The model under review builds one solid part; all positions refer to its coordinate system, in mm. A direction names the side the tool comes from. Round coordinates to 2 decimals unless told otherwise and drop trailing zeros. Loops run counter-clockwise (first coordinate to the right, second up) from the corner with the lowest first, then second, coordinate; pieces in that order, holes last. Notation, with made-up numbers: (13.25, 52.25) - (30.25, 52.25) arc R21 ccw to (30.25, 77.25) - close; hole circle Ø5 at (23, 50). An arc over 180 degrees is marked (long way). Answer as CSV lines item,"result".
from build123d import *
from build123d.topology import SkipClean

# Parameters (mm, degrees)
BOSS_EXTRUDE1_DEPTH = 3
SKETCH2_R           = 1.5
CUT_EXTRUDE1_DEPTH  = 9.507546276
CUT_EXTRUDE2_DEPTH  = 9.507546276


with BuildPart() as part:
    # Sketch1 → Boss-Extrude1 (new body)
    with BuildSketch(Plane(origin=(0, 0, 0), x_dir=(1, 0, 0), z_dir=(0, 1, 0))):
        with BuildLine():
            Line((-4.905, 2.614492754), (4.905, 2.614492754))
            ThreePointArc((4.905, 2.614492754), (7.519492754, 0), (4.905, -2.614492754))
            Line((4.905, -2.614492754), (-4.905, -2.614492754))
            ThreePointArc((-4.905, -2.614492754), (-7.519492754, 0), (-4.905, 2.614492754))
        make_face()
    extrude(amount=BOSS_EXTRUDE1_DEPTH)

    # Sketch2 → Cut-Extrude1 (cut, through all)
    with BuildSketch(Plane(origin=(0, 3, 0), x_dir=(1, 0, 0), z_dir=(0, 1, 0))):
        with Locations(Location((-4.905, 0, 0), (0, 0, 270))):
            Circle(SKETCH2_R)
        with Locations(Location((4.905, 0, 0), (0, 0, 270))):
            Circle(SKETCH2_R)
    extrude(amount=-CUT_EXTRUDE1_DEPTH, mode=Mode.SUBTRACT)

    # Sketch3 → Cut-Extrude2 (cut, through all)
    with SkipClean():  # the faces are left unmerged after this step: merging them gives an invalid solid
        with BuildSketch(Plane(origin=(0, 3, 0), x_dir=(1, 0, 0), z_dir=(0, 1, 0))):
            with BuildLine():
                Line((-2.666010862, 1.35), (2.666010862, 1.35))
                ThreePointArc((2.666010862, 1.35), (3.619308135, 2.276525596), (4.905, 2.614492754))
                Line((4.905, 2.614492754), (-4.905, 2.614492754))
                ThreePointArc((-4.905, 2.614492754), (-3.619308135, 2.276525596), (-2.666010862, 1.35))
            make_face()
            with BuildLine():
                Line((-2.666010862, -1.35), (2.666010862, -1.35))
                ThreePointArc((2.666010862, -1.35), (3.619308135, -2.276525596), (4.905, -2.614492754))
                Line((4.905, -2.614492754), (-4.905, -2.614492754))
                ThreePointArc((-4.905, -2.614492754), (-3.619308135, -2.276525596), (-2.666010862, -1.35))
            make_face()
        extrude(amount=-CUT_EXTRUDE2_DEPTH, mode=Mode.SUBTRACT)


solid = part.part
1. Take a section at D-D (x = 2.25). State the section outline as (y, z) points.
Numbers:
outline,"(0, -1.35) - (3, -1.35) - (3, 1.35) - (0, 1.35) - close"
2. Tool access review of faces 5 (the face through (0, 3, 0)), 6 (the face through (0, 2, -1.35)): name each direction out of +Z, -Z, +X, -X, +Y, -Y from which nothing blocks a thin tool from reaching the whole face with its end or side.
Numbers:
face 5,"+Z, -Z, +X, -X, +Y"
face 6,"-Z, +Y, -Y"
3. Take a section at A-A (x = -5.25). State the section outline as (y, z) points.
Numbers:
outline,"(0, -2.59) - (3, -2.59) - (3, -1.46) - (0, -1.46) - close; (0, 1.46) - (3, 1.46) - (3, 2.59) - (0, 2.59) - close"
4. Take a section at B-B (z = 0). State the section outline as (x, y) points (1 decimal), plus the area to 3 significant figures.
Numbers:
outline,"(-7.5, 0) - (-6.4, 0) - (-6.4, 3) - (-7.5, 3) - close; (-3.4, 0) - (3.4, 0) - (3.4, 3) - (-3.4, 3) - close; (6.4, 0) - (7.5, 0) - (7.5, 3) - (6.4, 3) - close"
area,"27.1 mm²"
5. Take a section at C-C (y = 0.9). State how many separate pieces and enclosed holes the cut face has, plus the area to 3 significant figures.
Numbers:
separate pieces,"1"
enclosed holes,"2"
area,"41.8 mm²"
6. Wall thickness on probe 1 along X at (y, z) = (1.7, 0) (1 decimal); probe 2 along X at (y, z) = (0.35, 0.4); probe 3 along Z at (x, y) = (1, 1.45): over which ranges is each line inside the solid? List them lowest first.
Numbers:
probe 1,"x = -7.5 to -6.4, -3.4 to 3.4, 6.4 to 7.5"
probe 2,"x = -7.49 to -6.35, -3.46 to 3.46, 6.35 to 7.49"
probe 3,"z = -1.35 to 1.35"
7. Draft analysis for pull direction Z (two halves, no side actions). For faces 1 (the face through (6.39, 1.52, -0.2)), 2 (the face through (-6.37, 1.52, -0.33)), 3 (the face through (0, 0, 0)), 4 (the face through (0, 2, 1.35)), state which applies: +Z half, -Z half, draft (parallel to the pull), parting line (faces both ways), or undercut.
Numbers:
face 1,"undercut"
face 2,"undercut"
face 3,"draft"
face 4,"+Z half"
8. Clearance check with flat-ended pins moving along their axes: pin 1 (3 mm diameter, centred on x = 5, z = 2, fed in from -Y); pin 2 (1 mm diameter, centred on x = 0, y = 1.5, fed in from +Z); pin 3 (1 mm diameter, centred on x = 6, y = 1, fed in from +Z). State where each tip first meets the part, or that it passes through.
Numbers:
pin 1,"stops at y = 0"
pin 2,"stops at z = 1.35"
pin 3,"stops at z = 2.55"
